Part model, mm, in its own coordinate system. A direction names the side the tool comes from. Give positions to 0.01 mm unless a question says otherwise; leave off trailing zeros. Loops run counter-clockwise (first coordinate to the right, second up) from the corner with the lowest first, then second, coordinate; pieces in that order, holes last. Notation, with made-up numbers: (-23, 29.25) -> (-19, 29.25) arc R23 cw to (-19, 38.25) -> close; hole circle Ø4 at (0, -33.5). An arc over 180 degrees is marked (long way). Write item = value, one per line.
from build123d import *
from build123d.topology import SkipClean

# Parameters (mm, degrees)
SKETCH1_W           = 28.25
SKETCH1_H           = 20.5
SKETCH1_R           = 2.5
BOSS_EXTRUDE1_DEPTH = 7.46
CUT_EXTRUDE2_DEPTH  = 1.1
SKETCH5_R           = 1
SKETCH5_R_2         = 3.62054265
CUT_EXTRUDE3_DEPTH  = 26.331790304
SKETCH6_R           = 3.05
CUT_EXTRUDE4_DEPTH  = 0.7
CUT_EXTRUDE5_START  = -0.7
SKETCH7_R           = 3.05
CUT_EXTRUDE5_DEPTH  = 0.7


with BuildPart() as part:
    # Sketch1 → Boss-Extrude1 (new body)
    with BuildSketch(Plane(origin=(0, 0, 0), x_dir=(1, 0, 0), z_dir=(0, 1, 0))):
        with Locations((-4.875, 5.25)):
            Rectangle(SKETCH1_W, SKETCH1_H)
        with Locations(Location((5.25, 11.75, 0), (0, 0, 90))):
            Circle(SKETCH1_R, mode=Mode.SUBTRACT)
        with Locations(Location((-10.75, 11.75, 0), (0, 0, 90))):
            Circle(SKETCH1_R, mode=Mode.SUBTRACT)
    extrude(amount=BOSS_EXTRUDE1_DEPTH)

    # Sketch3 → Cut-Extrude2 (cut)
    with BuildSketch(Plane(origin=(0, 7.46, 0), x_dir=(1, 0, 0), z_dir=(0, 1, 0))):
        with BuildLine():
            Line((-14.965459534, 2.114048767), (-0.367096675, 3.601884106))
            ThreePointArc((-0.367096675, 3.601884106), (3.62054265, 0), (-0.367096675, -3.601884106))
            Line((-0.367096675, -3.601884106), (-14.965459534, -2.114048767))
            ThreePointArc((-14.965459534, -2.114048767), (-16.875, 0), (-14.965459534, 2.114048767))
        make_face()
    extrude(amount=-CUT_EXTRUDE2_DEPTH, mode=Mode.SUBTRACT)

    # Sketch5 → Cut-Extrude3 (cut, through all)
    with SkipClean():  # the faces are left unmerged after this step: merging them gives an invalid solid
        with BuildSketch(Plane(origin=(0, 6.36, 0), x_dir=(1, 0, 0), z_dir=(0, 1, 0))):
            with Locations(Location((-12.6, 0, 0), (0, 0, 270))):
                Circle(SKETCH5_R)
            with Locations(Location((-6.5, 0, 0), (0, 0, 270))):
                Circle(SKETCH5_R)
            with Locations(Location((0, 0, 0), (0, 0, 270))):
                Circle(SKETCH5_R_2)
        extrude(amount=-CUT_EXTRUDE3_DEPTH, mode=Mode.SUBTRACT)

    # Sketch6 → Cut-Extrude4 (cut)
    with SkipClean():  # the faces are left unmerged after this step: merging them gives an invalid solid
        with BuildSketch(Plane(origin=(0, 7.46, 0), x_dir=(1, 0, 0), z_dir=(0, 1, 0))):
            with Locations(Location((-10.75, 11.75, 0), (0, 0, 270))):
                Circle(SKETCH6_R)
            with Locations(Location((5.25, 11.75, 0), (0, 0, 270))):
                Circle(SKETCH6_R)
        extrude(amount=-CUT_EXTRUDE4_DEPTH, mode=Mode.SUBTRACT)

    # Sketch7 → Cut-Extrude5 (cut)
    with SkipClean():  # the faces are left unmerged after this step: merging them gives an invalid solid
        with BuildSketch(Plane.XZ.offset(CUT_EXTRUDE5_START)):
            with Locations(Location((5.25, -11.75, 0), (0, 0, 90))):
                Circle(SKETCH7_R)
            with Locations(Location((-10.75, -11.75, 0), (0, 0, 90))):
                Circle(SKETCH7_R)
        extrude(amount=CUT_EXTRUDE5_DEPTH, mode=Mode.SUBTRACT)


solid = part.part
1) Pull direction Z, two halves, no side cores. Call faces 4 (the face through (-8, 6.76, -12)), 5 (the face through (-5, 4, -15.5)), 6 (the face through (-5, 0, -5)), 7 (the face through (-9, 6.36, 0)): pulls with the +Z half, pulls with the -Z half, needs draft (parallel to the pull), parting line crosses it, or undercut.
Resolved:
face_4 = undercut
face_5 = pulls with the -Z half
face_6 = needs draft
face_7 = undercut
2) Drop flat-ended pins along their axis: P1, Ø6, axis at x = 0, z = 0, coming from the -Y side; P2, Ø2, axis at x = -9.5, z = -1.5, coming from the +Y side. Give the stop position or say it passes through.
Resolved:
P1 = through
P2 = 6.36
3) Drill centre lines: line 1 along X through (y, z) = (2, 0); line 2 along X through (y, z) = (3, -11.75); line 3 along X through (y, z) = (7.3, -11.75). Where is each one in solid material? Low to high. Write a range as [from, to].
Resolved:
line_1 = [-19, -13.6], [-11.6, -7.5], [-5.5, -3.62], [3.62, 9.25]
line_2 = [-19, -13.25], [-8.25, 2.75], [7.75, 9.25]
line_3 = [-19, -13.8], [-7.7, 2.2], [8.3, 9.25]
4) Slice it at B-B, the plane z = 0. List the corners of the cut face in (x, y) (3 decimals).
Resolved:
outline = (-19, 0) -> (-13.6, 0) -> (-13.6, 6.36) -> (-16.875, 6.36) -> (-16.875, 7.46) -> (-19, 7.46) -> close; (-11.6, 0) -> (-7.5, 0) -> (-7.5, 6.36) -> (-11.6, 6.36) -> close; (-5.5, 0) -> (-3.621, 0) -> (-3.621, 6.36) -> (-5.5, 6.36) -> close; (3.621, 0) -> (9.25, 0) -> (9.25, 7.46) -> (3.621, 7.46) -> close
5) Slice it at C-C, the plane x = 0. List the corners of the cut face in (y, z), and give its area (3 significant figures).
Resolved:
outline = (0, -15.5) -> (7.46, -15.5) -> (7.46, -3.62) -> (0, -3.62) -> close; (0, 3.62) -> (7.46, 3.62) -> (7.46, 5) -> (0, 5) -> close
area = 98.9 mm²
6) Slice it at D-D, the plane y = 5.5. List the corners of the cut face in (x, z).
Resolved:
outline = (-19, -15.5) -> (9.25, -15.5) -> (9.25, 5) -> (-19, 5) -> close; hole circle Ø2 at (-12.6, 0); hole circle Ø5 at (-10.75, -11.75); hole circle Ø2 at (-6.5, 0); hole circle Ø7.24 at (0, 0); hole circle Ø5 at (5.25, -11.75)
7) Slice it at A-A, the plane z = -11.75. List the corners of the cut face in (x, y), and give its area (3 significant figures).
Resolved:
outline = (-19, 0) -> (-13.8, 0) -> (-13.8, 0.7) -> (-13.25, 0.7) -> (-13.25, 6.76) -> (-13.8, 6.76) -> (-13.8, 7.46) -> (-19, 7.46) -> close; (-8.25, 0.7) -> (-7.7, 0.7) -> (-7.7, 0) -> (2.2, 0) -> (2.2, 0.7) -> (2.75, 0.7) -> (2.75, 6.76) -> (2.2, 6.76) -> (2.2, 7.46) -> (-7.7, 7.46) -> (-7.7, 6.76) -> (-8.25, 6.76) -> close; (7.75, 0.7) -> (8.3, 0.7) -> (8.3, 0) -> (9.25, 0) -> (9.25, 7.46) -> (8.3, 7.46) -> (8.3, 6.76) -> (7.75, 6.76) -> close
area = 133 mm²
8) Which spindle directions (+Z, -Z, +X, -X, +Y, -Y) get a long thin tool onto all of the face, cutting with end or side? Do faces 1 (the face through (7.106, 0.355, -14.17)), 2 (the face through (-5.51, 3.22, -0.13)), 3 (the face through (-7.768, 6.918, -2.848)). Say none if no direction does.
Resolved:
face_1 = -Y
face_2 = +Y, -Y
face_3 = +Y
